For this review, take the finished solid that the model builds, in its own axes (mm). Coordinates: 2 decimals unless noted, no trailing zeros. Loops run counter-clockwise (first coordinate to the right, second up) from the corner with the lowest first, then second, coordinate; pieces in that order, holes last. Notation, with made-up numbers: M 10.5,-0.75 L 42.5,-0.75 A26 ccw 42.5,25.25 Z; hole C 89.25,6 d5. An arc over 180 degrees is marked long. Write item = value, one per line.
Autodesk Inventor part; units mm, degrees
ref_plane "YZ Plane" through (0, 0, 0) normal (1, 0, 0) x (0, 1, 0)
ref_plane "XZ Plane" through (0, 0, 0) normal (0, 1, 0) x (-1, 0, 0)
ref_plane "XY Plane" through (0, 0, 0) normal (0, 0, 1) x (1, 0, 0)
sketch "Sketch1" plane through (0, 0, 0) normal (0, 0, 1) x (1, 0, 0)
  line L0 (-40, 32.5) -> (40, 32.5)
  line L1 (40, 32.5) -> (40, -32.5)
  line L2 (40, -32.5) -> (-40, -32.5)
  line L3 (-40, -32.5) -> (-40, 32.5)
  line L4 (-40, 32.5) -> (40, -32.5) construction
  line L5 (40, 32.5) -> (-40, -32.5) construction
  line L6 (-8, 32.5) -> (-8, 24.5)
  line L7 (-8, 24.5) -> (-20, 24.5)
  line L8 (-20, 24.5) -> (-20, 28.5)
  line L9 (-20, 28.5) -> (-40, 28.5)
  line L10 (-40, -27) -> (-19, -27)
  line L11 (-19, -27) -> (-15.5, -23.5)
  line L12 (-15.5, -23.5) -> (-9.5, -23.5)
  line L13 (-9.5, -23.5) -> (-9.5, -32.5)
  line L14 (9.5, -32.5) -> (9.5, -23.5)
  line L15 (9.5, -23.5) -> (15.5, -23.5)
  line L16 (15.5, -23.5) -> (19, -27)
  line L17 (19, -27) -> (40, -27)
  point P0 (0, 0)
  dimension "d0" = 80
  dimension "d1" = 65
  dimension "d2" = 19
  dimension "d3" = 45
  dimension "d4" = 9
  dimension "d5" = 3.5
  dimension "d6" = 6
  dimension "d7" = 45
  dimension "d8" = 8
  dimension "d9" = 8
  dimension "d10" = 12
  dimension "d11" = 4
extrude "Extrusion1" add sketch "Sketch1" along normal blind 1.3 contours L0 L1 L17 L16 L15 L14 L2 L13 L12 L11 L10 L3 L9 L8 L7 L6
sketch "Sketch2" plane through (0, 0, 1.3) normal (0, 0, 1) x (1, 0, 0)
  line L0 (-35.7, -4.3) -> (35.7, -4.3) construction
  line L1 (-40, -27) -> (-19, -27)
  point P0 (0, 0)
  point P1 (0, -4.3)
  dimension "d14" = 71.4
  dimension "d15" = 22.7
hole "Hole1" at (-35.7, -4.3, 1.3) at (35.7, -4.3, 1.3) direction (0, 0, -1) diameter 2.5 end through all
sketch "Sketch4" plane through (-8, 32.5, 0) normal (0, 1, 0) x (1, 0, 0)
  line L0 (10.9, -2.9) -> (5.1, -2.9) construction
  line L1 (10.9, -1.3) -> (5.1, -1.3)
  line L2 (5.1, -4.5) -> (10.9, -4.5)
  arc A0 (10.9, -4.5) -> (10.9, -1.3) centre (10.9, -2.9) ccw
  arc A1 (5.1, -1.3) -> (5.1, -4.5) centre (5.1, -2.9) ccw
  line L3 (48, -1.3) -> (0, -1.3)
  line L4 (10.9, -2.9) -> (5.1, -2.9) construction
  line L5 (10.9, -1.7) -> (5.1, -1.7)
  line L6 (5.1, -4.1) -> (10.9, -4.1)
  arc A2 (10.9, -4.1) -> (10.9, -1.7) centre (10.9, -2.9) ccw
  arc A3 (5.1, -1.7) -> (5.1, -4.1) centre (5.1, -2.9) ccw
  point P0 (8, 0)
  point P1 (8, -2.9)
  point P2 (3.5, -2.9)
  point P3 (12.5, -2.9)
  point P4 (8, -2.9)
  dimension "d23" = 3.2
  dimension "d24" = 9
  dimension "d25" = 0.4
extrude "Extrusion2" add sketch "Sketch4" against normal blind 6.8
sketch "Sketch5" plane through (0, 0, 1.3) normal (0, 0, 1) x (1, 0, 0)
  circle A0 centre (-34.4, 23.1) radius 1.7
  circle A1 centre (34.4, 23.1) radius 1.7
  circle A2 centre (0, -22.3) radius 1.7
  line L0 (-34.4, 23.1) -> (34.4, 23.1) construction
  circle A3 centre (35.7, -4.3) radius 1.25
  point P0 (0, 0)
  point P1 (0, 23.1)
  dimension "d28" = 3.4
  dimension "d29" = 68.8
  dimension "d30" = 27.4
  dimension "d31" = 18
extrude "Extrusion3" add sketch "Sketch5" along normal blind 0.4 contours A0 | A1 | A2
equation "\"d7\" = d3"
properties part number "BDM-030"
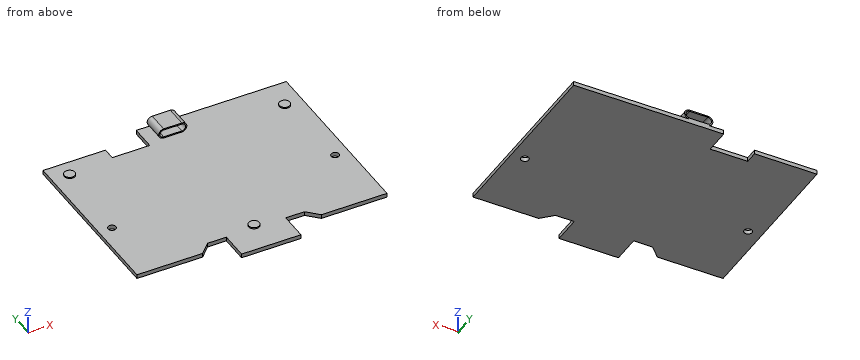
Q1. Add section C-C (y = -22.3). Write out the cut boundary in (x, z), and give its area (3 significant figures).
Solved:
outline = M -40,0 L 40,0 L 40,1.3 L 1.7,1.3 L 1.7,1.7 L -1.7,1.7 L -1.7,1.3 L -40,1.3 Z
area = 105 mm²
Q2. For pin 1 Ø3 at (x, y) = (35.7, -4.3) entering from +Z; pin 2 Ø1.4 at (y, z) = (-30, 1) entering from +X; pin 3 Ø1 at (x, z) = (12.5, 0.5) entering from -Y, all flat-tipped, find the tip position at first contact; note any pin that passes through.
Solved:
pin_1 = 1.3
pin_2 = 9.5
pin_3 = -23.5
Q3. Add section B-B (x = 0). Write out the cut boundary in (y, z).
Solved:
outline = M -32.5,0 L 32.5,0 L 32.5,1.7 L 25.7,1.7 L 25.7,1.3 L -20.6,1.3 L -20.6,1.7 L -24,1.7 L -24,1.3 L -32.5,1.3 Z; M 25.7,4.1 L 32.5,4.1 L 32.5,4.5 L 25.7,4.5 Z
Q4. Add section A-A (z = 2.9). Write out the cut boundary in (x, y), and give its area (3 significant figures).
Solved:
outline = M -4.5,25.7 L -4.1,25.7 L -4.1,32.5 L -4.5,32.5 Z; M 4.1,25.7 L 4.5,25.7 L 4.5,32.5 L 4.1,32.5 Z
area = 5.44 mm²
Q5. Add section D-D (x = 27). Write out the cut boundary in (y, z), and give its area (4 significant figures).
Solved:
outline = M -27,0 L 32.5,0 L 32.5,1.3 L -27,1.3 Z
area = 77.35 mm²
Q6. For line 1 along Y through (x, z) = (-35.7, 0.35); line 2 along Y through (x, z) = (35.7, 0.35); line 3 along X through (y, z) = (-4.3, 1.05), list the stretches that pass through material, from the lowest coordinate up.
Solved:
line_1 = -27 to -5.55, -3.05 to 28.5
line_2 = -27 to -5.55, -3.05 to 32.5
line_3 = -40 to -36.95, -34.45 to 34.45, 36.95 to 40
